Part model, mm, in its own coordinate system. Coordinates: 2 decimals unless noted, no trailing zeros. Loops run counter-clockwise (first coordinate to the right, second up) from the corner with the lowest first, then second, coordinate; pieces in that order, holes last. Notation, with made-up numbers: M -16.75,56.5 L 19.25,56.5 A14 ccw 19.25,79.5 Z; hole C -28.75,12.5 d4. An arc over 180 degrees is marked long. Use a Markdown table: item, result. Add a question column.
1) Band-saw the part on C-C (z = 4.75). List the corners of the cut face in (x, y), plus the area to 3 significant figures.
2) Band-saw the part on D-D (y = -9.85). List the corners of the cut face in (x, z), plus the area to 3 significant figures.
3) Wall check: probe 1 along X at (y, z) = (-9.85, 4.75); probe 2 along X at (y, z) = (5, 4); probe 3 along Y at (x, z) = (0, 4.25). Give the ranges that are in metal, low to high. Write a range as from..to.
4) Band-saw the part on A-A (x = 0). List the corners of the cut face in (y, z).
5) Band-saw the part on B-B (x = 102.5). List the corners of the cut face in (y, z), plus the area to 3 significant figures.
6) Pin check, flat tips, straight feed: pin 1 Ø3 at (y, z) = (29, 1) entering from -X; pin 2 Ø2 at (x, z) = (72, 1) entering from +Y. Stop position of each tip, or through.
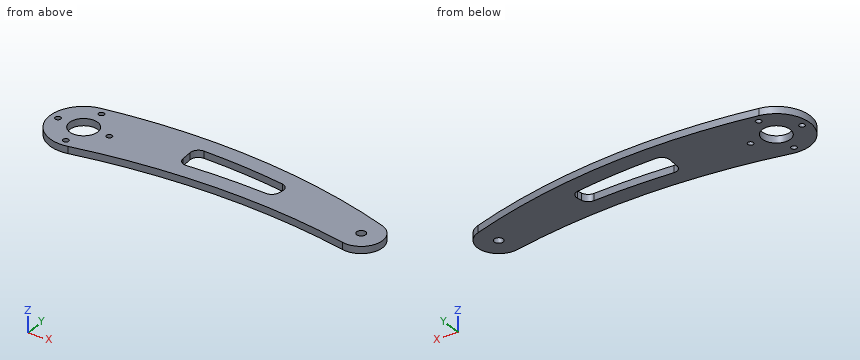
from build123d import *

# Parameters (mm, degrees)
SKETCH1_R           = 4
SKETCH1_R_2         = 2.5
SKETCH1_R_3         = 12.5
BOSS_EXTRUDE1_DEPTH = 6.2


with BuildPart() as part:
    # Sketch1 → Boss-Extrude1 (new body)
    with BuildSketch(Plane.XY):
        with BuildLine():
            ThreePointArc((-4.843381354, 29.606446208), (-29.489039073, -5.513308858), (6.180402599, -29.356474988))
            ThreePointArc((6.180402599, -29.356474988), (128.63005147, -16.382678773), (251.170355628, -28.47026553))
            ThreePointArc((251.170355628, -28.47026553), (273.303133895, -14.765534175), (260.982883768, 8.166778664))
            ThreePointArc((260.982883768, 8.166778664), (129.376669821, 35.090841966), (-4.843381354, 29.606446208))
        make_face()
        with Locations(Location((254.95, -9.85, 0), (0, 0, 180))):
            Circle(SKETCH1_R, mode=Mode.SUBTRACT)
        with Locations(Location((0, 23, 0), (0, 0, 180))):
            Circle(SKETCH1_R_2, mode=Mode.SUBTRACT)
        with Locations(Location((0, -23, 0), (0, 0, 180))):
            Circle(SKETCH1_R_2, mode=Mode.SUBTRACT)
        with Locations(Location((-23, 0, 0), (0, 0, 180))):
            Circle(SKETCH1_R_2, mode=Mode.SUBTRACT)
        with Locations(Location((23, 0, 0), (0, 0, 180))):
            Circle(SKETCH1_R_2, mode=Mode.SUBTRACT)
        with Locations(Location((0, 0, 0), (0, 0, 180))):
            Circle(SKETCH1_R_3, mode=Mode.SUBTRACT)
        with BuildLine():
            Line((85.299988347, 14.334161591), (86.047515876, 3.894174942))
            ThreePointArc((86.047515876, 3.894174942), (88.416575223, -0.870831987), (93.451584576, -2.593160073))
            ThreePointArc((93.451584576, -2.593160073), (129.051714651, -1.468455886), (164.657677356, -2.390215498))
            ThreePointArc((164.657677356, -2.390215498), (169.415573807, -0.864394835), (171.943987902, 3.445225739))
            Line((171.943987902, 3.445225739), (172.629734019, 7.547504331))
            ThreePointArc((172.629734019, 7.547504331), (171.396804828, 12.804877005), (166.788880257, 15.62038992))
            ThreePointArc((166.788880257, 15.62038992), (129.692411097, 20.014503602), (92.380913243, 21.833400801))
            ThreePointArc((92.380913243, 21.833400801), (87.192448356, 19.639856576), (85.299988347, 14.334161591))
        make_face(mode=Mode.SUBTRACT)
    extrude(amount=BOSS_EXTRUDE1_DEPTH)


solid = part.part
Entries:
| question | item | result |
|---|---|---|
| 1 | outline | M -4.84,29.61 A30 ccw long 6.18,-29.36 A605 cw 251.17,-28.47 A19 ccw 260.98,8.17 A555 ccw Z; hole C -23,0 d5; hole C 0,0 d25; hole C 0,-23 d5; hole C 0,23 d5; hole C 23,0 d5; hole M 85.3,14.33 L 86.05,3.89 A7 ccw 93.45,-2.59 A619.91 cw 164.66,-2.39 A7 ccw 171.94,3.45 L 172.63,7.55 A7 ccw 166.79,15.62 A540 ccw 92.38,21.83 A7 ccw Z; hole C 254.95,-9.85 d8 |
| 1 | area | 12,600 mm2 |
| 2 | outline | M -28.34,0 L -7.7,0 L -7.7,6.2 L -28.34,6.2 Z; M 7.7,0 L 250.95,0 L 250.95,6.2 L 7.7,6.2 Z; M 258.95,0 L 273.95,0 L 273.95,6.2 L 258.95,6.2 Z |
| 2 | area | 1,730 mm2 |
| 3 | probe 1 | -28.34..-7.7, 7.7..250.95, 258.95..273.95 |
| 3 | probe 2 | -29.58..-11.46, 11.46..85.97, 172.2..266.8 |
| 3 | probe 3 | -30..-25.5, -20.5..-12.5, 12.5..20.5, 25.5..30.38 |
| 4 | outline | M -30,0 L -25.5,0 L -25.5,6.2 L -30,6.2 Z; M -20.5,0 L -12.5,0 L -12.5,6.2 L -20.5,6.2 Z; M 12.5,0 L 20.5,0 L 20.5,6.2 L 12.5,6.2 Z; M 25.5,0 L 30.38,0 L 30.38,6.2 L 25.5,6.2 Z |
| 5 | outline | M -17.04,0 L -2.11,0 L -2.11,6.2 L -17.04,6.2 Z; M 21.6,0 L 36.6,0 L 36.6,6.2 L 21.6,6.2 Z |
| 5 | area | 186 mm2 |
| 6 | pin 1 | x = -11.99 |
| 6 | pin 2 | y = 36.76 |
